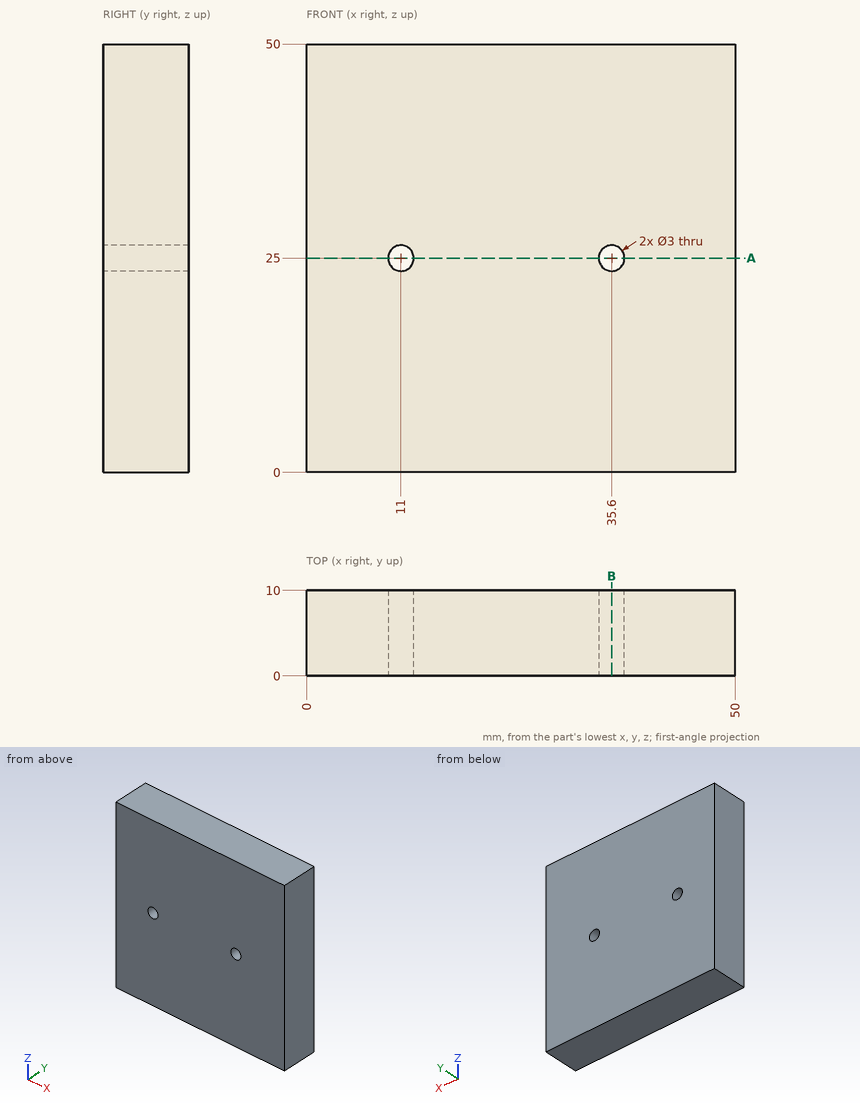
Source: three-view drawing plus pictorial views. Frame: mm from the lowest corner of the part. Give positions to 0.01 mm unless a question says otherwise; leave off trailing zeros. Order: outer loops, then holes, each group sorted by start corner. A loop starts at its lowest first (then second) coordinate and runs counter-clockwise, first axis right, second up. Notation, with made-up numbers: (-34, 75) - (8, 75) arc R35 cw to (8, 111) - close; hole circle Ø10 at (-39, -5). An arc over 180 degrees is marked (long way). Put each result on its own line as item: value.
Item 1: Contact query for a flat-ended pin moving along its axis: pin 1 (3 mm diameter, centred on y = 4.5, z = 18.5, fed in from -X). Output: stop coordinate, or through.
Found:
pin 1: stops at x = 0
Item 2: Section query B-B, the plane x = 35.6. Return loops of the section in (y, z).
Found:
outline: (0, 0) - (10, 0) - (10, 23.5) - (0, 23.5) - close; (0, 26.5) - (10, 26.5) - (10, 50) - (0, 50) - close
Item 3: Ray query, L1, parallel to Z at x = 11, y = 6. Return the intervals inside material, ascending. Write a range as from..to.
Found:
L1: z = 0..23.5, 26.5..50
Item 4: Section query A-A, the plane z = 25. Return loops of the section in (x, y), then the cut area to 3 significant figures.
Found:
outline: (0, 0) - (9.5, 0) - (9.5, 10) - (0, 10) - close; (12.5, 0) - (34.1, 0) - (34.1, 10) - (12.5, 10) - close; (37.1, 0) - (50, 0) - (50, 10) - (37.1, 10) - close
area: 440 mm^2
